Geometry: final body of the model. Coordinates: model frame, mm. A direction names the side the tool comes from. Give positions to 0.01 mm unless a question says otherwise; leave off trailing zeros. Loops run counter-clockwise (first coordinate to the right, second up) from the corner with the lowest first, then second, coordinate; pieces in that order, holes last. Notation, with made-up numbers: M 89,-13.75 L 100,-13.75 A20 cw 100,3.25 Z; hole C 70.5,88 d1. An arc over 180 degrees is marked long. One line per question, with ' | ' between items. Start each with the question number.
from build123d import *

# Parameters (mm, degrees)
SKETCH_1_R          = 25
EXTRUDE_1_DEPTH     = 30
FILLET_1_R          = 4
FILLET_2_R          = 4
SKETCH_2_R          = 17.5
EXTRUDE_2_DEPTH     = 2
FILLET_3_R          = 2
EXTRUDE_START       = 2
SKETCH_3_R          = 17.5
EXTRUDE_3_DEPTH     = 2
FILLET_4_R          = 2
SKETCH_4_R          = 4.2
CUT_EXTRUDE_1_DEPTH = 50.050993874


with BuildPart() as part:
    # 草图1 → 凸台-拉伸1 (new body)
    with BuildSketch(Plane.XY):
        Circle(SKETCH_1_R)
    extrude(amount=EXTRUDE_1_DEPTH)

    # 圆角1
    fillet_1_edges = [part.edges().sort_by_distance(p)[0] for p in [
        (-25, 0, 30),
    ]]
    fillet(fillet_1_edges, radius=FILLET_1_R)

    # 圆角2
    fillet_2_edges = [part.edges().sort_by_distance(p)[0] for p in [
        (-25, 0, 0),
    ]]
    fillet(fillet_2_edges, radius=FILLET_2_R)

    # 草图2 → 凸台-拉伸2 (add)
    with BuildSketch(Plane.XY.offset(30)):
        Circle(SKETCH_2_R)
    extrude(amount=EXTRUDE_2_DEPTH)

    # 圆角3
    fillet_3_edges = [part.edges().sort_by_distance(p)[0] for p in [
        (-17.5, 0, 32),
    ]]
    fillet(fillet_3_edges, radius=FILLET_3_R - 0.0001)  # a hair under: the kernel refuses the full size

    # 草图3 → 凸台-拉伸3 (add)
    with BuildSketch(Plane(origin=(0, 0, 0), x_dir=(-1, 0, 0), z_dir=(0, 0, -1)).offset(EXTRUDE_START)):
        with Locations(Location((0, 0, 0), (0, 0, 180))):
            Circle(SKETCH_3_R)
    extrude(amount=-EXTRUDE_3_DEPTH)

    # 圆角4
    fillet_4_edges = [part.edges().sort_by_distance(p)[0] for p in [
        (-17.5, 0, -2),
    ]]
    fillet(fillet_4_edges, radius=FILLET_4_R - 0.0001)  # a hair under: the kernel refuses the full size

    # 草图4 → 切除-拉伸1 (cut, through all)
    with BuildSketch(Plane(origin=(0, 0, -2), x_dir=(-1, 0, 0), z_dir=(0, 0, -1))):
        Circle(SKETCH_4_R)
    extrude(amount=-CUT_EXTRUDE_1_DEPTH, mode=Mode.SUBTRACT)


solid = part.part
Q1. Draft query along X for faces 1 (the flat face through (3.2, 3.2, -2)), 2 (the cylindrical face through (-4.006, 1.262, 14.762)), 3 (the cylindrical face through (23.846, 7.509, 14.846)). Return one class per face: released by +X, released by -X, zero draft, split by the parting line, or undercut.
Q2. Material intervals for L1, parallel to Y at x = 0, z = 20; L2, parallel to Z at x = -18, y = 4.5; L3, parallel to Z at x = 7, y = -14, sorted ascending.
Q3. Set-up query: faces 4 (the flat face through (-8, 16, 30)), 5 (the flat face through (3.2, -3.2, 32)), 6 (the flat face through (-8, 16, 0)). Return all of +Z, -Z, +X, -X, +Y, -Y with unobstructed straight access to the full face (end or side cutting, diameter ignored); none if empty.
Q4. Contact query for flat-ended pins moving along their axis: pin 1 (1 mm diameter, centred on y = -15, z = 4.5, fed in from +X); pin 2 (6 mm diameter, centred on x = 11.5, z = 14.5, fed in from -Y); pin 3 (1 mm diameter, centred on x = 16, y = -3, fed in from -Z); pin 4 (6.5 mm diameter, centred on x = 0, y = 0, fed in from -Z). Output: stop coordinate, or through.
Q5. Section C-C, the plane z = 1.5. Output: boundary loops of the cut face in (x, y) (1 decimal), plus the area to 3 significant figures.
Model answer:
1) face 1: zero draft | face 2: undercut | face 3: split by the parting line
2) L1: y = -25 to -4.2, 4.2 to 25 | L2: z = 0 to 30 | L3: z = -1.99 to 31.99
3) face 4: +Z | face 5: +Z, +X, -X, +Y, -Y | face 6: -Z
4) pin 1: stops at x = 20.37 | pin 2: stops at y = -23.51 | pin 3: stops at z = -1.98 | pin 4: passes through
5) outline: C 0,0 d48.2; hole C 0,0 d8.4 | area: 1,770 mm^2
